```python
from build123d import *

# Parameters (mm, degrees)
SKETCH_W        = 10
SKETCH_H        = 10
SKETCH_R        = 1.65
PAD_DEPTH       = 4
SKETCH001_W     = 10
SKETCH001_H     = 24
PAD001_DEPTH    = 8
SKETCH002_W     = 6
SKETCH002_H     = 20
POCKET_DEPTH    = 9
SKETCH003_W     = 4
SKETCH003_H     = 20
POCKET001_DEPTH = 5


with BuildPart() as part:
    # Sketch → Pad (new body)
    with BuildSketch(Plane.XY):
        with Locations((-5, 0)):
            Rectangle(SKETCH_W, SKETCH_H)
        with Locations((-5, 0)):
            Circle(SKETCH_R, mode=Mode.SUBTRACT)
    extrude(amount=PAD_DEPTH)

    # Sketch001 → Pad001 (join)
    with BuildSketch(Plane.YZ):
        with Locations((-0.02241, 12)):
            Rectangle(SKETCH001_W, SKETCH001_H)
    extrude(amount=PAD001_DEPTH)

    # Sketch002 (on Face11 of Pad001) → Pocket (cut)
    with BuildSketch(Plane.XZ.offset(5.02241)):
        with Locations((4, 12)):
            Rectangle(SKETCH002_W, SKETCH002_H)
    extrude(amount=-POCKET_DEPTH, mode=Mode.SUBTRACT)

    # Sketch003 (on Face18 of Pocket) → Pocket001 (cut)
    with BuildSketch(Plane.XZ.offset(-3.97759)):
        with Locations((4, 12)):
            Rectangle(SKETCH003_W, SKETCH003_H)
    extrude(amount=-POCKET001_DEPTH, mode=Mode.SUBTRACT)


solid = part.part
```
Geometry: final body of the model. Coordinates: model frame, mm. A direction names the side the tool comes from. Give positions to 0.01 mm unless a question says otherwise; leave off trailing zeros. Loops run counter-clockwise (first coordinate to the right, second up) from the corner with the lowest first, then second, coordinate; pieces in that order, holes last. Notation, with made-up numbers: (45.5, -13) -> (80.5, -13) arc R12 cw to (80.5, 3) -> close; hole circle Ø4 at (64, 69.5). An arc over 180 degrees is marked (long way). Use CSV: the item, a comma, the result in double quotes.
(1) Cut plane B-B (y = 0). Output: boundary loops of the cut face in (x, z), plus the area to 3 significant figures.
From the geometry:
outline,"(-10, 0) -> (-6.65, 0) -> (-6.65, 4) -> (-10, 4) -> close; (-3.35, 0) -> (8, 0) -> (8, 24) -> (0, 24) -> (0, 4) -> (-3.35, 4) -> close; hole (1, 2) -> (7, 2) -> (7, 22) -> (1, 22) -> close"
area,"98.8 mm^2"
(2) Cut plane A-A (z = 2.5). Count the separate pieces of the cut face and the enclosed holes in it, plus the area to 3 significant figures.
From the geometry:
separate pieces,"2"
enclosed holes,"1"
area,"113 mm^2"
(3) Ray query, line 1 along X through (y, z) = (0, 10); line 2 along Z through (x, y) = (2.75, -3); line 3 along Y through (x, z) = (-5, 2.55). Return the intervals inside material, ascending. Write a range as [from, to].
From the geometry:
line 1,"[0, 1], [7, 8]"
line 2,"[0, 2], [22, 24]"
line 3,"[-5, -1.65], [1.65, 5]"
(4) Pull-direction query (Y, two-part tool) for faces 1 (the face through (1.5, 3.978, 12.1)), 2 (the face through (1, -1, 12)), 3 (the face through (-6.65, 0.07, 1.97)), 4 (the face through (7, 4.978, 12)); classes: released by +Y, released by -Y, zero draft, split by the parting line, or undercut.
From the geometry:
face 1,"released by -Y"
face 2,"zero draft"
face 3,"undercut"
face 4,"released by +Y"
(5) Cut plane D-D (z = 13.25). Output: boundary loops of the cut face in (x, y).
From the geometry:
outline,"(0, -5.02) -> (1, -5.02) -> (1, 3.98) -> (2, 3.98) -> (2, 4.98) -> (0, 4.98) -> close; (6, 3.98) -> (7, 3.98) -> (7, -5.02) -> (8, -5.02) -> (8, 4.98) -> (6, 4.98) -> close"
(6) Access query for faces 5 (the face through (-5, 2, 4)), 6 (the face through (4, 0, 22)), 7 (the face through (6, 4.5, 11.9)), 8 (the face through (-1, 0, 0)), 9 (the face through (-5, -5, 2)). Directions: +Z, -Z, +X, -X, +Y, -Y. A direction counts if a zero-diameter tool reaches every point of the face in a straight line with its end or side. Return the directions, or none.
From the geometry:
face 5,"+Z, -X, +Y, -Y"
face 6,"-Y"
face 7,"+Y, -Y"
face 8,"-Z, +X, -X, +Y, -Y"
face 9,"+Z, -Z, -X, -Y"
(7) First-contact query: P1, Ø0.8, axis at x = 1.5, z = 9.5, coming from the -Y side; P2, Ø4.5, axis at y = -2.5, z = 16.5, coming from the -X side; P3, Ø4.5, axis at x = -2.5, z = 2, coming from the -Y side. Flat tips, straight axial feed; report the tip coordinate or a pass-through.
From the geometry:
P1,"y = 3.98"
P2,"x = 0"
P3,"y = -5"
(8) Cut plane C-C (x = 4.5). Output: boundary loops of the cut face in (y, z).
From the geometry:
outline,"(-5.02, 0) -> (4.98, 0) -> (4.98, 2) -> (-5.02, 2) -> close; (-5.02, 22) -> (4.98, 22) -> (4.98, 24) -> (-5.02, 24) -> close"
